Design review of the part shown in the three views and the two pictorial views. Dimensions are in mm from the part's minimum x, y and z. A direction names the side the tool comes from. Round coordinates to 2 decimals unless told otherwise and drop trailing zeros. Write each loop counter-clockwise with the first axis right and the second up, starting at its lowest first coordinate (ties: lowest second). Pieces come first, ordered by that corner, then holes. Notation, with made-up numbers: (-40, 20.5) -> (6, 20.5) arc R9 ccw to (6, 32.5) -> close; hole circle Ø2 at (88, 43). An arc over 180 degrees is marked (long way). Answer as a JSON object with one key per item and string values. Group by question number.
1) We need section A-A, the plane y = 34.5. Write out the cut boundary in (x, z), then the cut area to 3 significant figures.
2) To check wall thickness, follow probe 1 along X at (y, z) = (44, 53); probe 2 along Z at (x, y) = (31, 34); probe 3 along Y at (x, z) = (32.8, 63). State the ranges of each line that lie inside material, in increasing order. Write a range as [from, to].
3) We need section D-D, the plane y = 22. Write out the cut boundary in (x, z), then the cut area to 3 significant figures.
4) Machinability: for the marked faces 1, 2 and 3, which of the approach directions +Z, -Z, +X, -X, +Y, -Y give a long, thin tool a straight path to every point of the face, cutting with its end or side? Answer none if there is none.
5) Insertion check: pin 1 Ø0.8 at (y, z) = (33.5, 0.5) entering from -X; pin 2 Ø3 at (y, z) = (19, 29) entering from -X; pin 3 Ø1.8 at (x, y) = (6.4, 44.5) entering from -Z; pin 4 Ø1 at (x, y) = (20, 61.5) entering from -Z. Each pin has a flat end and moves straight along its axis. Give the tip position at first contact, or say it passes through.
6) We need section B-B, the plane x = 26.4. Write out the cut boundary in (y, z).
7) We need section C-C, the plane z = 63. Write out the cut boundary in (x, y), then the cut area to 3 significant figures.
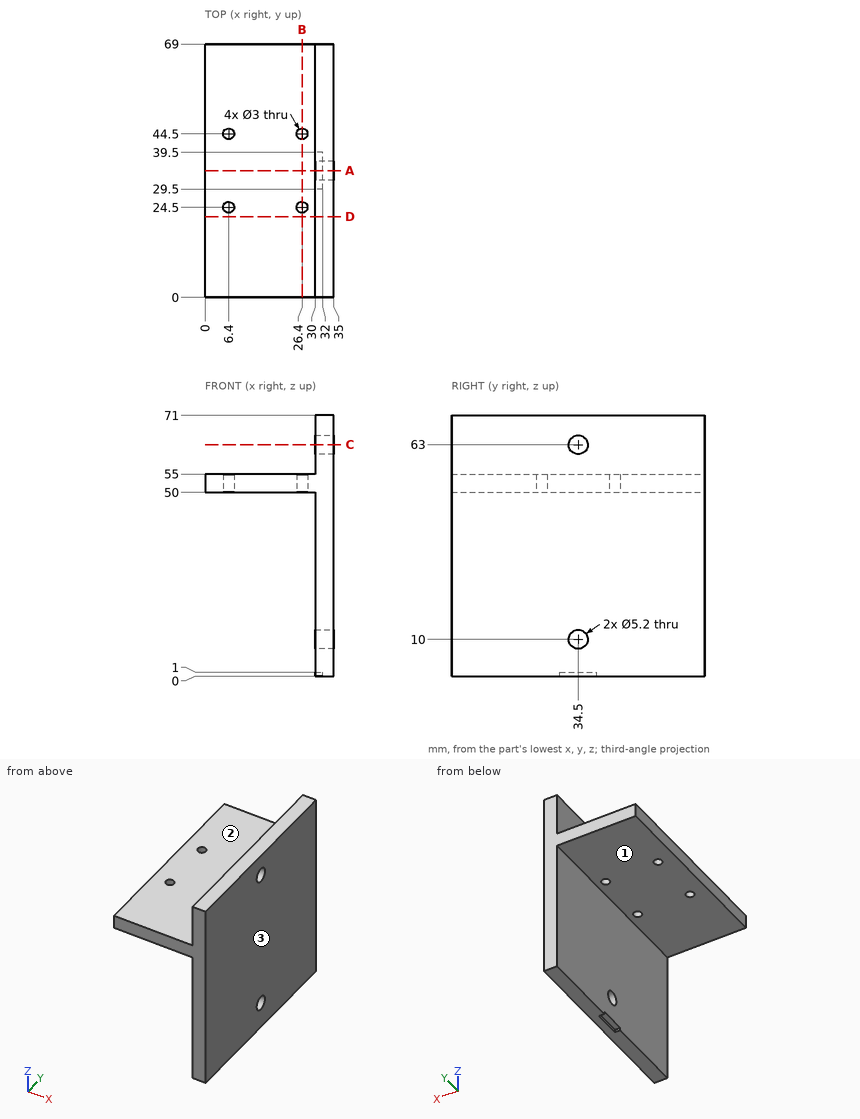
Here are the results:
{
 "1": {"outline": "(0, 50) -> (30, 50) -> (30, 12.6) -> (35, 12.6) -> (35, 60.4) -> (30, 60.4) -> (30, 55) -> (0, 55) -> close; (30, 1) -> (32, 1) -> (32, 0) -> (35, 0) -> (35, 7.4) -> (30, 7.4) -> close; (30, 65.6) -> (35, 65.6) -> (35, 71) -> (30, 71) -> close", "area": "451 mm^2"},
 "2": {"probe 1": "x = [0, 4.99], [7.81, 24.99], [27.81, 35]", "probe 2": "z = [1, 7.45], [12.55, 60.45], [65.55, 71]", "probe 3": "y = [0, 31.9], [37.1, 69]"},
 "3": {"outline": "(0, 50) -> (30, 50) -> (30, 0) -> (35, 0) -> (35, 71) -> (30, 71) -> (30, 55) -> (0, 55) -> close", "area": "505 mm^2"},
 "4": {"face 1": "-Z, -X, +Y, -Y", "face 2": "+Z, -X, +Y, -Y", "face 3": "+Z, -Z, +X, +Y, -Y"},
 "5": {"pin 1": "stops at x = 32", "pin 2": "stops at x = 30", "pin 3": "passes through", "pin 4": "stops at z = 50"},
 "6": {"outline": "(0, 50) -> (23, 50) -> (23, 55) -> (0, 55) -> close; (26, 50) -> (43, 50) -> (43, 55) -> (26, 55) -> close; (46, 50) -> (69, 50) -> (69, 55) -> (46, 55) -> close"},
 "7": {"outline": "(30, 0) -> (35, 0) -> (35, 31.9) -> (30, 31.9) -> close; (30, 37.1) -> (35, 37.1) -> (35, 69) -> (30, 69) -> close", "area": "319 mm^2"}
}
